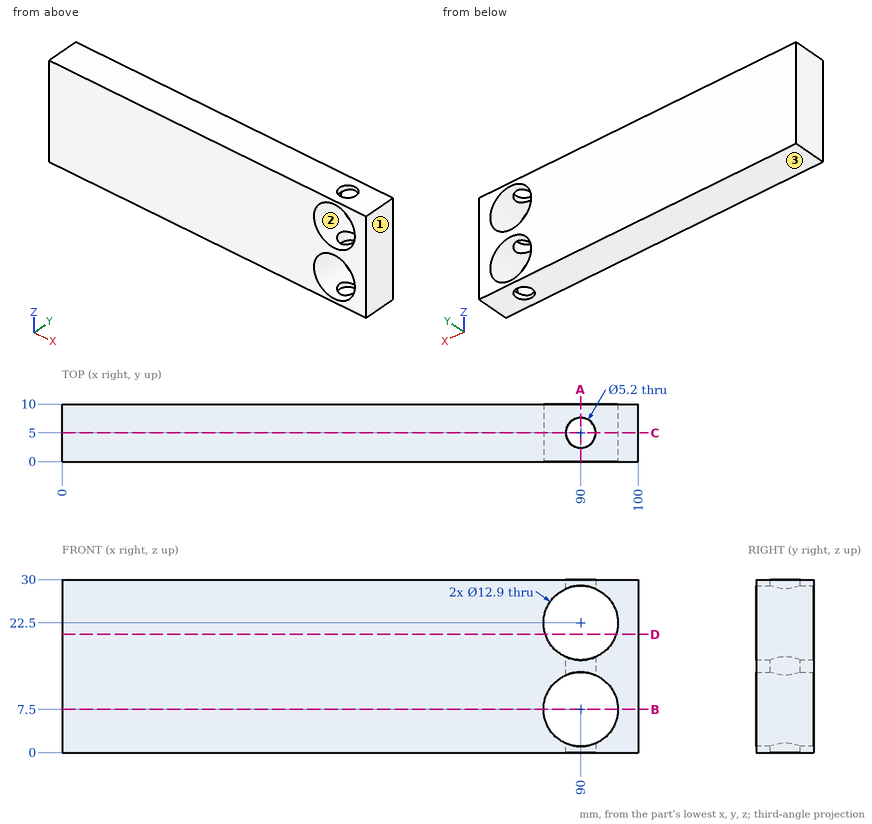
Part print with two shaded views. Sizes in mm from the minimum x, y, z corner. Round coordinates to 2 decimals unless told otherwise and drop trailing zeros. Order: outer loops, then holes, each group sorted by start corner. A loop starts at its lowest first (then second) coordinate and runs counter-clockwise, first axis right, second up. Notation, with made-up numbers: (42, -22.75) - (73, -22.75) arc R11 ccw to (73, -7.75) - close; hole circle Ø7 at (11, 82.25). An arc over 180 degrees is marked (long way). Return JSON: item names as keys, results as strings.
(1) Cut at A-A (x = 90). Give the cut face in (y, z).
Answer key:
{"outline": "(0, 0) - (2.4, 0) - (2.4, 1.05) - (0, 1.05) - close; (0, 13.95) - (2.4, 13.95) - (2.4, 16.05) - (0, 16.05) - close; (0, 28.95) - (2.4, 28.95) - (2.4, 30) - (0, 30) - close; (7.6, 0) - (10, 0) - (10, 1.05) - (7.6, 1.05) - close; (7.6, 13.95) - (10, 13.95) - (10, 16.05) - (7.6, 16.05) - close; (7.6, 28.95) - (10, 28.95) - (10, 30) - (7.6, 30) - close"}
(2) Cut at C-C (y = 5). Give the cut face in (x, z).
Answer key:
{"outline": "(0, 0) - (87.4, 0) - (87.4, 1.6) arc R6.45 cw to (87.4, 13.4) - (87.4, 16.6) arc R6.45 cw to (87.4, 28.4) - (87.4, 30) - (0, 30) - close; (92.6, 0) - (100, 0) - (100, 30) - (92.6, 30) - (92.6, 28.4) arc R6.45 cw to (92.6, 16.6) - (92.6, 13.4) arc R6.45 cw to (92.6, 1.6) - close"}
(3) Cut at D-D (z = 20.5). Give the cut face in (x, y).
Answer key:
{"outline": "(0, 0) - (83.87, 0) - (83.87, 10) - (0, 10) - close; (96.13, 0) - (100, 0) - (100, 10) - (96.13, 10) - close"}
(4) Wall check: probe 1 along Y at (x, z) = (90, 0.85); probe 2 along X at (y, z) = (1, 8.5); probe 3 along X at (y, z) = (4.25, 26.5). Give the ranges that are in metal, low to high. Write a range as from..to.
Answer key:
{"probe 1": "y = 0..2.4, 7.6..10", "probe 2": "x = 0..83.63, 96.37..100", "probe 3": "x = 0..84.94, 95.06..100"}
(5) Cut at B-B (z = 7.5). Give the cut face in (x, y).
Answer key:
{"outline": "(0, 0) - (83.55, 0) - (83.55, 10) - (0, 10) - close; (96.45, 0) - (100, 0) - (100, 10) - (96.45, 10) - close"}
(6) Pull direction X, two halves, no side cores. Call the marked faces 1, 2 and 3: +X half, -X half, draft (parallel to the pull), parting line (faces both ways), or undercut.
Answer key:
{"face 1": "+X half", "face 2": "undercut", "face 3": "draft"}
